```python
from build123d import *

# Parameters (mm, degrees)
F2_SIZE = 0.5
F3_R    = 1


with BuildPart() as f1:
    # F0 (on Front) → F1 (revolve)
    with BuildSketch(Plane.XZ):
        Polygon((0, 13.5), (-1.5, 13.5), (-1.5, 2), (-2.35, 2), (-2.35, 0), (0, 0), align=None)
    revolve(axis=Axis((0, 0, 3.320783), (0, 0, -1)))

    # F2
    f2_edges = [f1.edges().sort_by_distance(p)[0] for p in [
        (1.5, 0, 13.5),
    ]]
    chamfer(f2_edges, length=F2_SIZE)

    # F3
    f3_edges = [f1.edges().sort_by_distance(p)[0] for p in [
        (2.35, 0, 0),
    ]]
    fillet(f3_edges, radius=F3_R)


solid = f1.part
```
CAD build for the part. Positions are in the model's coordinates, mm. A direction names the side the tool comes from. Give positions to 0.01 mm unless a question says otherwise; leave off trailing zeros. Write each loop counter-clockwise with the first axis right and the second up, starting at its lowest first coordinate (ties: lowest second). Pieces come first, ordered by that corner, then holes. Notation, with made-up numbers: (-20, -15.5) -> (13, -15.5) arc R18 cw to (13, -2.5) -> close; hole circle Ø6 at (41.25, 56). An arc over 180 degrees is marked (long way). Write each question's results on one line, items separated by ' | '.
1. Which spindle directions (+Z, -Z, +X, -X, +Y, -Y) get a long thin tool onto all of the face, cutting with end or side? Do faces 1 (the cylindrical face through (1.5, 0.07, 7.42)), 2 (the flat face through (0, 0, 0)). Say none if no direction does.
Geometry check:
face 1: +Z | face 2: -Z, +X, -X, +Y, -Y
2. Cut at C-C, the plane z = 1.75. Write the cut outline in (x, y).
Geometry check:
outline: circle Ø4.7 at (0, 0)
3. Cut at A-A, the plane x = 0. Write the cut outline in (y, z).
Geometry check:
outline: (-2.35, 1) arc R1 ccw to (-1.35, 0) -> (1.35, 0) arc R1 ccw to (2.35, 1) -> (2.35, 2) -> (1.5, 2) -> (1.5, 13) -> (1, 13.5) -> (-1, 13.5) -> (-1.5, 13) -> (-1.5, 2) -> (-2.35, 2) -> close
4. Drop flat-ended pins along their axis: P1, Ø1, axis at x = -1, z = 10.5, coming from the +Y side; P2, Ø1.5, axis at x = 2, y = -1.5, coming from the +Z side; P3, Ø1.5, axis at y = 0.5, z = 9.5, coming from the +X side. Give the stop position or say it passes through.
Geometry check:
P1: y = 1.41 | P2: z = 2 | P3: x = 1.5
5. Wall check: probe 1 along X at (y, z) = (1.05, 8.5); probe 2 along X at (y, z) = (-0.4, 10); probe 3 along Z at (x, y) = (0.6, -1.1). Give the ranges that are in metal, low to high. Write a range as [from, to].
Geometry check:
probe 1: [-1.07, 1.07] | probe 2: [-1.45, 1.45] | probe 3: [0, 13.25]
